Part model, mm, in its own coordinate system. A direction names the side the tool comes from. Round coordinates to 2 decimals unless told otherwise and drop trailing zeros. Order: outer loops, then holes, each group sorted by start corner. A loop starts at its lowest first (then second) coordinate and runs counter-clockwise, first axis right, second up. Notation, with made-up numbers: M 11,-30.75 L 17,-30.75 A14 ccw 17,-6.75 Z; hole C 48.25,6 d4. An arc over 180 degrees is marked long. Write each question's results on one line, items separated by ' | '. Start each with the question number.
1. Probe L1, parallel to Z at x = -24, y = -5.25; L2, parallel to X at y = -5.75, z = -15.5; L3, parallel to Z at x = 0, y = -3.5. List the from-to ranges inside material, lowest first. Write a range as [from, to].
2. Which spindle directions (+Z, -Z, +X, -X, +Y, -Y) get a long thin tool onto all of the face, cutting with end or side? Do faces 1 (the face through (32.117, -0.902, -10.392)), 2 (the face through (-30.62, -3.45, 21.28)), 3 (the face through (-33.156, -3.493, -21.952)). Say none if no direction does.
3. Band-saw the part on A-A, the plane x = 0. List the corners of the cut face in (y, z).
4. Two-plate mould, pull along Z, no slides. Class faces 4 (the face through (-7, 0, -10)), 5 (the face through (0, -3, 16.86)), 6 (the face through (0.041, -0.902, -33.757)): +Z half, -Z half, draft (parallel to the pull), parting line (faces both ways), or undercut.
5. Band-saw the part on B-B, the plane z = 2. Give the number of separate pieces and of enclosed holes in the cut face, then the cut area to 3 significant figures.
6. Drop flat-ended pins along their axis: pin 1 Ø2 at (x, y) = (-24, -5) entering from +Z; pin 2 Ø1.1 at (x, y) = (-1, -3.5) entering from -Z; pin 3 Ø4 at (y, z) = (-3.5, -5.5) entering from -X. Give the stop position or say it passes through.
```python
from build123d import *

# Parameters (mm, degrees)
F0_R     = 12.251715
F0_R_2   = 11.1
F1_DEPTH = 7
F2_R     = 3


with BuildPart() as f1:
    # F0 (on Front) → F1 (new body)
    with BuildSketch(Plane.XZ):
        Polygon((18.475209, 29.36019), (9.237604, 13.36019), (-9.237604, 13.36019), (-18.475209, 29.36019), (-22.214047, 26.643765), (-9.851719, 12.91401), (-15.560873, -4.656958), (-33.632353, -8.49817), (-32.204244, -12.893438), (-15.326302, -5.378893), (-0.379544, -16.238348), (-2.310729, -34.612348), (2.310729, -34.612348), (0.379544, -16.238348), (15.326302, -5.378893), (32.204244, -12.893438), (33.632353, -8.49817), (15.560873, -4.656958), (9.851719, 12.91401), (22.214047, 26.643765), align=None)
        Circle(F0_R, mode=Mode.SUBTRACT)
        Polygon((-9.237604, 13.36019), (9.237604, 13.36019), (18.475209, 29.36019), (9.237604, 45.36019), (-9.237604, 45.36019), (-18.475209, 29.36019), align=None)
        Polygon((14.433757, 29.36019), (7.216878, 16.86019), (-7.216878, 16.86019), (-14.433757, 29.36019), (-7.216878, 41.86019), (7.216878, 41.86019), align=None, mode=Mode.SUBTRACT)
        Polygon((40.285528, 22.802553), (22.214047, 26.643765), (9.851719, 12.91401), (15.560873, -4.656958), (33.632353, -8.49817), (45.994681, 5.231586), align=None)
        Polygon((13.804856, 12.073744), (23.462924, 22.800116), (37.581268, 19.799169), (42.041545, 6.071851), (32.383476, -4.654521), (18.265132, -1.653574), align=None, mode=Mode.SUBTRACT)
        Polygon((-9.851719, 12.91401), (-22.214047, 26.643765), (-40.285528, 22.802553), (-45.994681, 5.231586), (-33.632353, -8.49817), (-15.560873, -4.656958), align=None)
        Polygon((-18.265132, -1.653574), (-32.383476, -4.654521), (-42.041545, 6.071851), (-37.581268, 19.799169), (-23.462924, 22.800116), (-13.804856, 12.073744), align=None, mode=Mode.SUBTRACT)
        Polygon((34.13543, -31.267437), (32.204244, -12.893438), (15.326302, -5.378893), (0.379544, -16.238348), (2.310729, -34.612348), (19.188672, -42.126892), align=None)
        Polygon((15.748748, -9.398206), (28.934641, -15.268943), (30.44338, -29.62363), (18.766225, -38.10758), (5.580332, -32.236842), (4.071594, -17.882155), align=None, mode=Mode.SUBTRACT)
        Polygon((-15.326302, -5.378893), (-32.204244, -12.893438), (-34.13543, -31.267437), (-19.188672, -42.126892), (-2.310729, -34.612348), (-0.379544, -16.238348), align=None)
        Polygon((-4.071594, -17.882155), (-5.580332, -32.236842), (-18.766225, -38.10758), (-30.44338, -29.62363), (-28.934641, -15.268943), (-15.748748, -9.398206), align=None, mode=Mode.SUBTRACT)
        Circle(F0_R)
        Circle(F0_R_2, mode=Mode.SUBTRACT)
    extrude(amount=F1_DEPTH)

    # F2
    f2_edges = [f1.edges().sort_by_distance(p)[0] for p in [
        (0, -7, 45.36019),
        (13.856406, -7, 37.36019),
        (31.249787, -7, 24.723159),
        (20.344628, -7, 28.001978),
        (43.140104, -7, 14.01707),
        (39.813517, -7, -1.633292),
        (33.169837, -7, -22.080437),
        (32.918299, -7, -10.695804),
        (26.662051, -7, -36.697165),
        (10.7497, -7, -38.36962),
        (-10.7497, -7, -38.36962),
        (0, -7, -34.612348),
        (-26.662051, -7, -36.697165),
        (-33.169837, -7, -22.080437),
        (-32.918299, -7, -10.695804),
        (-43.140104, -7, 14.01707),
        (-39.813517, -7, -1.633292),
        (-31.249787, -7, 24.723159),
        (-20.344628, -7, 28.001978),
        (-13.856406, -7, 37.36019),
        (-26.662051, 0, -36.697165),
        (-10.7497, 0, -38.36962),
        (0, 0, -34.612348),
        (10.7497, 0, -38.36962),
        (26.662051, 0, -36.697165),
        (33.169837, 0, -22.080437),
        (39.813517, 0, -1.633292),
        (43.140104, 0, 14.01707),
        (31.249787, 0, 24.723159),
        (32.918299, 0, -10.695804),
        (20.344628, 0, 28.001978),
        (13.856406, 0, 37.36019),
        (0, 0, 45.36019),
        (-13.856406, 0, 37.36019),
        (-20.344628, 0, 28.001978),
        (-31.249787, 0, 24.723159),
        (-43.140104, 0, 14.01707),
        (-33.169837, 0, -22.080437),
        (-39.813517, 0, -1.633292),
        (-32.918299, 0, -10.695804),
    ]]
    fillet(f2_edges, radius=F2_R)


solid = f1.part
```
Solution:
1) L1: [-38.29, -34.31], [-13.07, -2.87], [22.69, 25.99] | L2: [-31.91, -28.96], [-7.35, 7.35], [28.96, 31.91] | L3: [-34.61, -11.1], [11.1, 16.86], [41.86, 45.36]
2) face 1: +X, +Y | face 2: +Y, -Y | face 3: -X, +Y, -Y
3) outline: M -7,-31.61 A3 ccw -4,-34.61 L -3,-34.61 A3 ccw 0,-31.61 L 0,-11.1 L -7,-11.1 Z; M -7,11.1 L 0,11.1 L 0,16.86 L -7,16.86 Z; M -7,41.86 L 0,41.86 L 0,42.36 A3 ccw -3,45.36 L -4,45.36 A3 ccw -7,42.36 Z
4) face 4: draft | face 5: undercut | face 6: -Z half
5) separate pieces: 4 | enclosed holes: 0 | area: 142 mm^2
6) pin 1: z = 26.41 | pin 2: z = -34.61 | pin 3: x = -38.13
